Design review of the part shown in the three views and the two pictorial views. Dimensions are in mm from the part's minimum x, y and z. Give positions to 0.01 mm unless a question says otherwise; leave off trailing zeros. Order: outer loops, then holes, each group sorted by start corner. A loop starts at its lowest first (then second) coordinate and runs counter-clockwise, first axis right, second up.
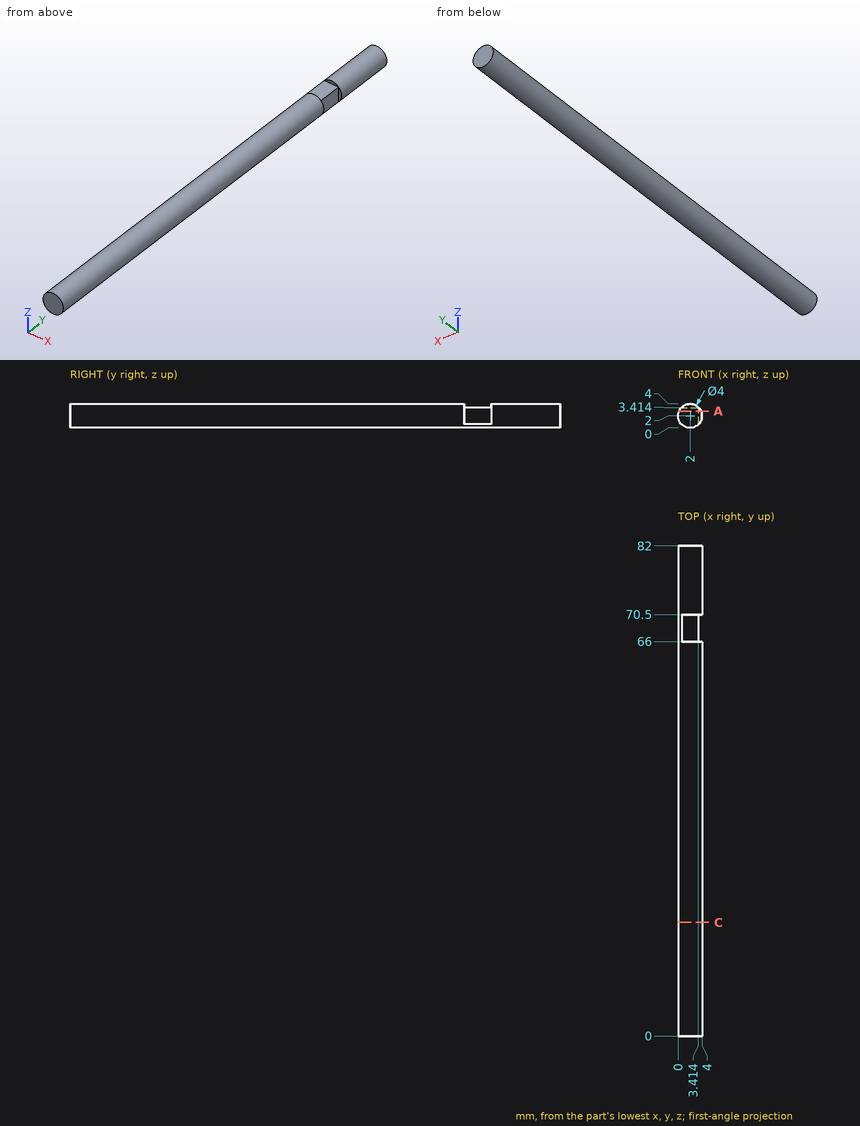
1) To check wall thickness, follow line 1 (X direction, y = 69.5, z = 0.6) (1 decimal); line 2 (Y direction, x = 3.75, z = 1.2); line 3 (Z direction, x = 0.6, y = 64.5). State the ranges of each line that lie inside material, in increasing order.
Answer sheet:
line 1: x = 0.6 to 3.4
line 2: y = 0 to 66, 70.5 to 82
line 3: z = 0.57 to 3.43
2) We need section A-A on z = 2.8. Give the boundary of the cut face in (x, y).
Answer sheet:
outline: (0.17, 0) - (3.83, 0) - (3.83, 66) - (3.41, 66) - (3.41, 70.5) - (3.83, 70.5) - (3.83, 82) - (0.17, 82) - close
3) We need section C-C on y = 19. Give the boundary of the cut face in (x, z), then the cut area to 3 significant figures.
Answer sheet:
outline: circle Ø4 at (2, 2)
area: 12.6 mm2
4) Clearance check with a flat-ended pin moving along its axis: pin 1 (0.8 mm diameter, centred on x = 2.5, y = 69, fed in from +Z). State where the tip first meets the part, or that it passes through.
Answer sheet:
pin 1: stops at z = 3.41
